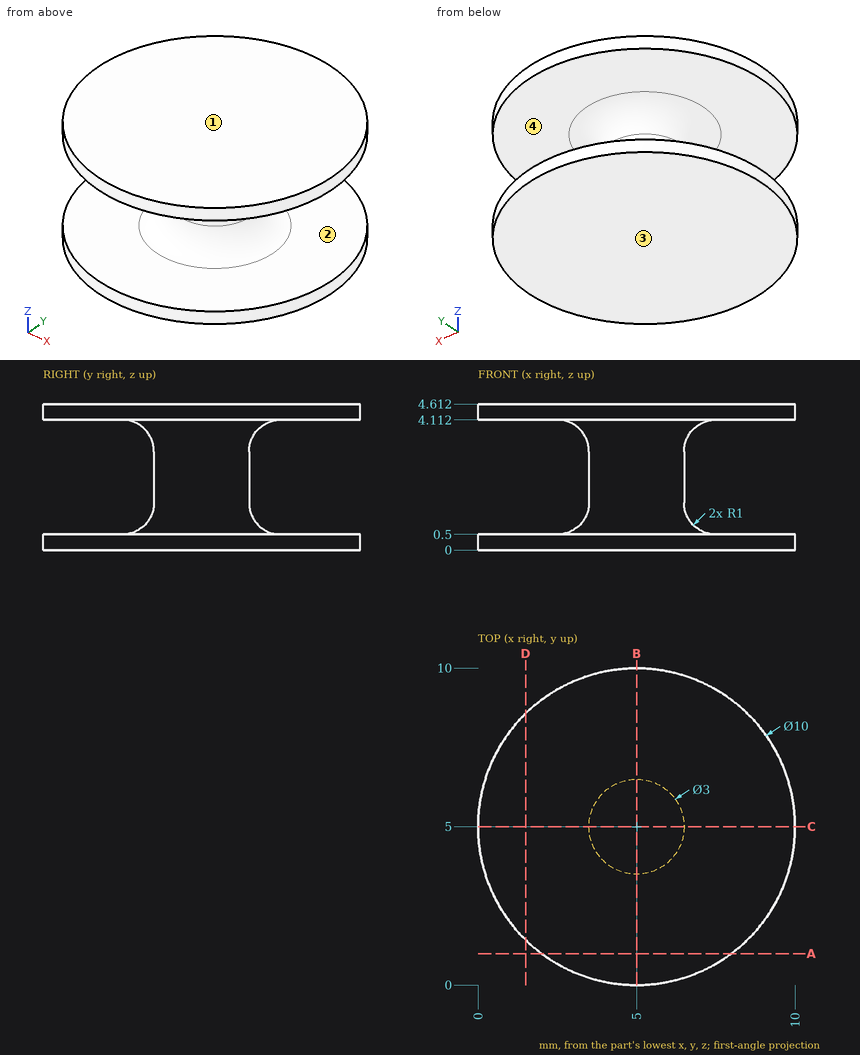
Answer from the drawing. Dimensions are ordinates in mm from the lowest x, y and z of the part. Give positions to 0.01 mm unless a question says otherwise; leave off trailing zeros. Write each loop counter-clockwise with the first axis right and the second up, starting at its lowest first coordinate (ties: lowest second). Pieces come first, ordered by that corner, then holes. Notation, with made-up numbers: (-15.5, 53) - (-0.5, 53) arc R22 ccw to (-0.5, 63) - close; hole circle Ø10 at (-34.5, -19). An arc over 180 degrees is marked (long way). Answer in a Markdown table with one row per item. Add a question column.
Item 1: Section A-A, the plane y = 1 is taken. Write down the section's boundary in (x, z).
Item 2: Find the intervals of material crossed by L1, parallel to Z at x = 8.5, y = 5.5; L2, parallel to Y at x = 5, z = 2.3; L3, parallel to Z at x = 5.5, y = 3.5 (1 decimal), in increasing order.
Item 3: Section D-D, the plane x = 1.5 is taken. Write down the section's boundary in (y, z).
Item 4: Section B-B, the plane x = 5 is taken. Write down the section's boundary in (y, z).
Item 5: Determine the mould class of the marked faces 1, 2, 3 and 4 for opening direction Z: pulls with the +Z half, pulls with the -Z half, needs draft (parallel to the pull), parting line crosses it, or undercut.
Recorded:
| question | item | result |
|---|---|---|
| 1 | outline | (2, 0) - (8, 0) - (8, 0.5) - (2, 0.5) - close; (2, 4.11) - (8, 4.11) - (8, 4.61) - (2, 4.61) - close |
| 2 | L1 | z = 0 to 0.5, 4.11 to 4.61 |
| 2 | L2 | y = 3.5 to 6.5 |
| 2 | L3 | z = 0 to 1.1, 3.5 to 4.6 |
| 3 | outline | (1.43, 0) - (8.57, 0) - (8.57, 0.5) - (1.43, 0.5) - close; (1.43, 4.11) - (8.57, 4.11) - (8.57, 4.61) - (1.43, 4.61) - close |
| 4 | outline | (0, 0) - (10, 0) - (10, 0.5) - (7.5, 0.5) arc R1 cw to (6.5, 1.5) - (6.5, 3.11) arc R1 cw to (7.5, 4.11) - (10, 4.11) - (10, 4.61) - (0, 4.61) - (0, 4.11) - (2.5, 4.11) arc R1 cw to (3.5, 3.11) - (3.5, 1.5) arc R1 cw to (2.5, 0.5) - (0, 0.5) - close |
| 5 | face 1 | pulls with the +Z half |
| 5 | face 2 | undercut |
| 5 | face 3 | pulls with the -Z half |
| 5 | face 4 | undercut |
